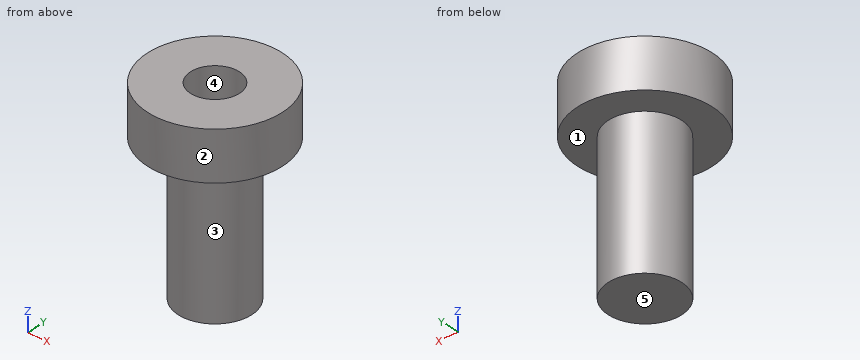
from build123d import *

# Parameters (mm, degrees)
F0_R     = 2.75
F1_DEPTH = 8
F2_R     = 2.75
F2_R_2   = 1.5
F3_DEPTH = 6
F4_R     = 1
F5_DEPTH = 2


with BuildPart() as f1:
    # F0 (on Top) → F1 (new body)
    with BuildSketch(Plane.XY):
        Circle(F0_R)
    extrude(amount=F1_DEPTH)

    # F2 (on face) → F3 (cut)
    with BuildSketch(Plane(origin=(0, 0, 0), x_dir=(1, 0, 0), z_dir=(0, 0, -1))):
        Circle(F2_R)
        Circle(F2_R_2, mode=Mode.SUBTRACT)
    extrude(amount=-F3_DEPTH, mode=Mode.SUBTRACT)

    # F4 (on face) → F5 (cut)
    with BuildSketch(Plane.XY.offset(8)):
        Circle(F4_R)
    extrude(amount=-F5_DEPTH, mode=Mode.SUBTRACT)


solid = f1.part
CAD build for the part. Positions are in the model's coordinates, mm. Face numbers are marked on the shaded views. A direction names the side the tool comes from. Coordinates: 2 decimals unless noted, no trailing zeros. Write each loop counter-clockwise with the first axis right and the second up, starting at its lowest first coordinate (ties: lowest second). Pieces come first, ordered by that corner, then holes. Notation, with made-up numbers: M -24.5,53 L 22.5,53 A24 cw 22.5,66 Z; hole C -34,23 d2. An arc over 180 degrees is marked long. Answer as a JSON object with one key per item and string values. Group by question number.
1) Pin check, flat tip, straight feed: pin 1 Ø1 at (x, z) = (-0.5, 3.5) entering from -Y. Stop position of the tip, or through.
2) Tool access for the marked faces 1 and 2: list every direction of +Z, -Z, +X, -X, +Y, -Y with a clear straight run to the whole face (end or side of a thin tool).
3) Saw through at A-A (y = 0). Write the cut outline in (x, z), plus the area to 3 significant figures.
4) Mould opens along Y. For the marked faces 3, 4 and 5 say: +Y half, -Y half, draft (parallel to the pull), parting line (faces both ways), or undercut.
5) Saw through at C-C (z = 4). Write the cut outline in (x, y), plus the area to 3 significant figures.
6) Wall check: line 1 (Y direction, x = 0, z = 7.25); line 2 (Z direction, x = -0.4, y = 2.05); line 3 (X direction, y = 0.05, z = 5.75). Give the ranges that are in metal, low to high. Write a range as from..to.
7) Saw through at D-D (y = -1.2). Write the cut outline in (x, z), plus the area to 3 significant figures.
Values follow:
{
 "1": {"pin 1": "stops at y = -1.5"},
 "2": {"face 1": "-Z", "face 2": "+Z, -Z"},
 "3": {"outline": "M -2.75,6 L -1.5,6 L -1.5,0 L 1.5,0 L 1.5,6 L 2.75,6 L 2.75,8 L 1,8 L 1,6 L -1,6 L -1,8 L -2.75,8 Z", "area": "25.0 mm2"},
 "4": {"face 3": "parting line", "face 4": "undercut", "face 5": "draft"},
 "5": {"outline": "C 0,0 d3", "area": "7.07 mm2"},
 "6": {"line 1": "y = -2.75..-1, 1..2.75", "line 2": "z = 6..8", "line 3": "x = -1.5..1.5"},
 "7": {"outline": "M -2.47,6 L -0.9,6 L -0.9,0 L 0.9,0 L 0.9,6 L 2.47,6 L 2.47,8 L -2.47,8 Z", "area": "20.7 mm2"}
}
